from build123d import *

# Parameters (mm, degrees)
BOSS_EXTRUDE1_DEPTH = 25.4
SKETCH2_R           = 3.175
CUT_EXTRUDE1_DEPTH  = 12.7
SKETCH3_R           = 3.175
BOSS_EXTRUDE2_DEPTH = 9.525


with BuildPart() as part:
    # Sketch1 → Boss-Extrude1 (new body)
    with BuildSketch(Plane(origin=(0, 0, 0), x_dir=(1, 0, 0), z_dir=(0, 1, 0))):
        Polygon((0, 5.499261314), (-4.7625, 2.749630657), (-4.7625, -2.749630657), (0, -5.499261314), (4.7625, -2.749630657), (4.7625, 2.749630657), align=None)
    extrude(amount=BOSS_EXTRUDE1_DEPTH)

    # Sketch2 → Cut-Extrude1 (cut)
    with BuildSketch(Plane.XZ):
        with Locations(Location((0, 0, 0), (0, 0, 270))):
            Circle(SKETCH2_R)
    extrude(amount=-CUT_EXTRUDE1_DEPTH, mode=Mode.SUBTRACT)

    # Sketch3 → Boss-Extrude2 (add)
    with BuildSketch(Plane(origin=(0, 25.4, 0), x_dir=(1, 0, 0), z_dir=(0, 1, 0))):
        with Locations(Location((0, 0, 0), (0, 0, 90))):
            Circle(SKETCH3_R)
    extrude(amount=BOSS_EXTRUDE2_DEPTH)


solid = part.part
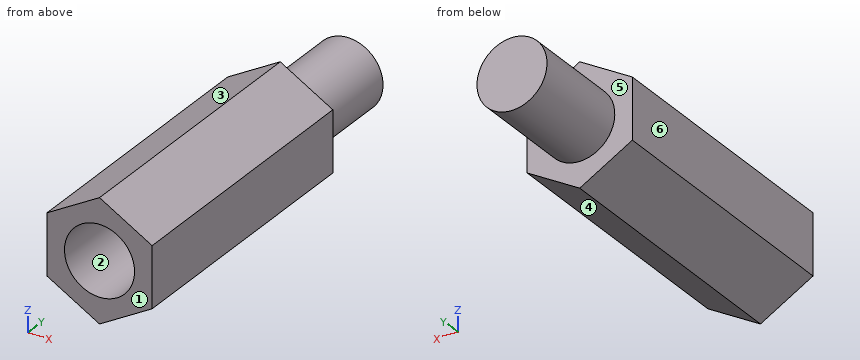
Model file for the job. Use its own axes, mm. Face numbers are marked on the shaded views. A direction names the side the tool comes from. Give positions to 0.01 mm unless a question says otherwise; leave off trailing zeros. Order: outer loops, then holes, each group sorted by start corner. A loop starts at its lowest first (then second) coordinate and runs counter-clockwise, first axis right, second up. Notation, with made-up numbers: (61, 16.25) -> (114, 16.25) arc R30 cw to (114, 47.25) -> close; hole circle Ø4 at (68.25, 88). An arc over 180 degrees is marked (long way). Use CSV: the item, a comma, the result in double quotes.
1. Band-saw the part on D-D, the plane x = 2.5. Give the cut face in (y, z) (3 decimals), then the cut area to 3 significant figures.
Outcome:
outline,"(0, -4.056) -> (25.4, -4.056) -> (25.4, -1.957) -> (34.925, -1.957) -> (34.925, 1.957) -> (25.4, 1.957) -> (25.4, 4.056) -> (0, 4.056) -> (0, 1.957) -> (12.7, 1.957) -> (12.7, -1.957) -> (0, -1.957) -> close"
area,"194 mm²"
2. 3-axis set-ups, long thin cutter, end or side, ignore diameter. For the marked faces 5 and 6: which of +Z, -Z, +X, -X, +Y, -Y reach the whole face in a straight line?
Outcome:
face 5,"+Y"
face 6,"+Z, -Z, -X, +Y, -Y"
3. Drill centre lines: line 1 along X through (y, z) = (4.75, 0) (1 decimal); line 2 along Y through (x, z) = (-1, -3.5); line 3 along Y through (x, z) = (-3, 0.75) (3 decimals). Where is each one in solid material? Low to high. Write a range as from..to.
Outcome:
line 1,"-4.8..-3.2, 3.2..4.8"
line 2,"0..25.4"
line 3,"12.7..34.925"
4. Mould opens along Z. For the marked faces 1, 2, 3 and 4 say: +Z half, -Z half, draft (parallel to the pull), parting line (faces both ways), or undercut.
Outcome:
face 1,"draft"
face 2,"undercut"
face 3,"+Z half"
face 4,"-Z half"
5. Band-saw the part on C-C, the plane z = 0. Give the cut face in (x, y) (1 decimal).
Outcome:
outline,"(-4.8, 0) -> (-3.2, 0) -> (-3.2, 12.7) -> (3.2, 12.7) -> (3.2, 0) -> (4.8, 0) -> (4.8, 25.4) -> (3.2, 25.4) -> (3.2, 34.9) -> (-3.2, 34.9) -> (-3.2, 25.4) -> (-4.8, 25.4) -> close"
6. Band-saw the part on B-B, the plane y = 20. Give the cut face in (x, z), then the cut area to 3 significant figures.
Outcome:
outline,"(-4.76, -2.75) -> (0, -5.5) -> (4.76, -2.75) -> (4.76, 2.75) -> (0, 5.5) -> (-4.76, 2.75) -> close"
area,"78.6 mm²"
7. Drop flat-ended pins along their axis: pin 1 (3 mm diameter, centred on y = 31, z = 2, fed in from -X); pin 2 (1.5 mm diameter, centred on y = 14, z = 4, fed in from +X); pin 3 (1 mm diameter, centred on x = -2, z = -0.5, fed in from -Y). Give the stop position or say it passes through.
Outcome:
pin 1,"x = -3.14"
pin 2,"x = 3.9"
pin 3,"y = 12.7"
